Build history of the part. All positions in model axes, mm. Face numbers are marked on the shaded views. A direction names the side the tool comes from. Round coordinates to 2 decimals unless told otherwise and drop trailing zeros. Order: outer loops, then holes, each group sorted by start corner. A loop starts at its lowest first (then second) coordinate and runs counter-clockwise, first axis right, second up. Notation, with made-up numbers: (33, 87.25) - (42, 87.25) arc R13 ccw to (42, 100.25) - close; hole circle Ø6 at (20, -21.5). An arc over 180 degrees is marked (long way). Write each question's results on one line, items separated by ' | '. Start each with the question number.
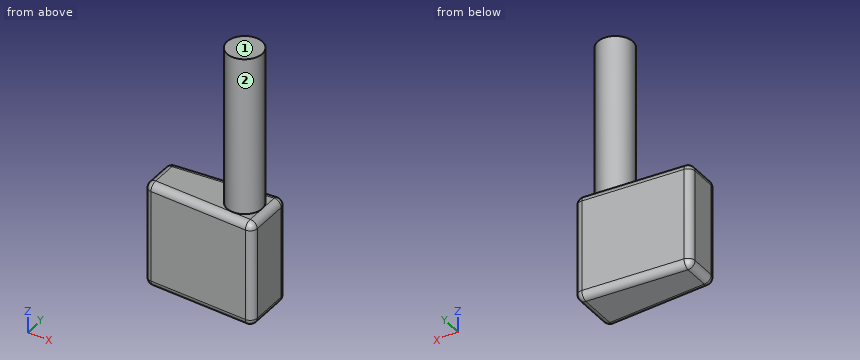
```python
from build123d import *

# Parameters (mm, degrees)
RESSALTO_EXTRUS_O1_DEPTH = 30
FILETE1_R                = 2
ESBO_O4_R                = 5
RESSALTO_EXTRUS_O2_DEPTH = 45


with BuildPart() as part:
    # Esboço2 → Ressalto-extrusão1 (new body)
    with BuildSketch(Plane.XY):
        Polygon((0, 0), (0, 15), (-32, 13), (-32, 2), align=None)
    extrude(amount=RESSALTO_EXTRUS_O1_DEPTH)

    # Filete1
    filete1_edges = [part.edges().sort_by_distance(p)[0] for p in [
        (-16, 14, 30),
        (-32, 7.5, 30),
        (-16, 1, 30),
        (-32, 7.5, 0),
        (-16, 14, 0),
        (0, 7.5, 0),
        (-16, 1, 0),
        (-32, 2, 15),
        (-32, 13, 15),
        (0, 15, 15),
        (0, 0, 15),
        (0, 7.5, 30),
    ]]
    fillet(filete1_edges, radius=FILETE1_R)

    # Esboço4 → Ressalto-extrusão2 (add)
    with BuildSketch(Plane.XY.offset(30)):
        with Locations((-7, 7.5)):
            Circle(ESBO_O4_R)
    extrude(amount=RESSALTO_EXTRUS_O2_DEPTH)


solid = part.part
```
1. Cut at C-C (z = 57). List the corners of the cut face in (x, y), plus the area to 3 significant figures.
2. Flat gauge pins, fed straight in: pin 1 Ø4 at (x, z) = (-20.5, 22) entering from -Y; pin 2 Ø4 at (x, z) = (-13.5, 20) entering from +Y; pin 3 Ø3 at (x, y) = (-23, 13.5) entering from -Z. Where does each tip first touch, or does it go through?
3. Cut at A-A (z = 9). List the corners of the cut face in (x, y), plus the area to 3 significant figures.
4. Wall check: line 1 (Z direction, x = -22, y = 11.75); line 2 (Y direction, x = -27.5, z = 7.5); line 3 (Z direction, x = -30.5, y = 8.25). Give the ranges that are in metal, low to high. Write a range as from..to.
5. Cut at B-B (y = 10). List the corners of the cut face in (x, z), plus the area to 3 significant figures.
6. 3-axis set-ups, long thin cutter, end or side, ignore diameter. For the marked faces 1 and 2: which of +Z, -Z, +X, -X, +Y, -Y reach the whole face in a straight line?
A:
1) outline: circle Ø10 at (-7, 7.5) | area: 78.5 mm^2
2) pin 1: stops at y = 1.16 | pin 2: stops at y = 14.28 | pin 3: stops at z = 0.05
3) outline: (-32, 3.88) arc R2 ccw to (-30.12, 1.88) - (-2.12, 0.13) arc R2 ccw to (0, 2.13) - (0, 12.87) arc R2 ccw to (-2.12, 14.87) - (-30.12, 13.12) arc R2 ccw to (-32, 11.12) - close | area: 413 mm^2
4) line 1: z = 0..30 | line 2: y = 1.72..13.28 | line 3: z = 0.06..29.94
5) outline: (-32, 2) arc R2 ccw to (-30, 0) - (-2, 0) arc R2 ccw to (0, 2) - (0, 28) arc R2 ccw to (-2, 30) - (-2.67, 30) - (-2.67, 75) - (-11.33, 75) - (-11.33, 30) - (-30, 30) arc R2 ccw to (-32, 28) - close | area: 1,350 mm^2
6) face 1: +Z, +X, -X, +Y, -Y | face 2: +Z
